Source: CAD feature listing. Evaluate the final solid. Frame: model axes, mm. Face numbers are marked on the shaded views. A direction names the side the tool comes from. Round coordinates to 2 decimals unless told otherwise and drop trailing zeros. Order: outer loops, then holes, each group sorted by start corner. A loop starts at its lowest first (then second) coordinate and runs counter-clockwise, first axis right, second up. Notation, with made-up numbers: M -33.5,-22.5 L 1.5,-22.5 A28 ccw 1.5,16.5 Z; hole C 58.5,61.5 d6. An arc over 180 degrees is marked long. Use one line per item in the form item = value. Start each with the question number.
Q1. Pull-direction query (X, two-part tool) for the marked faces 3, 4 and 5; classes: pulls with the +X half, pulls with the -X half, needs draft (parallel to the pull), parting line crosses it, or undercut.
Q2. Section C-C (z = 72). Return the cut outline in (x, y).
Q3. Material intervals for probe 1 along X at (y, z) = (-59.5, 29); probe 2 along Y at (x, z) = (-11, 73.5); probe 3 along Z at (x, y) = (16, 6.5), sorted ascending.
Q4. Section A-A (z = 35). Return the cut outline in (x, y), plus the area to 4 significant figures.
Q5. Section D-D (y = -66). Return the cut outline in (x, z), plus the area to 3 significant figures.
Q6. Contact query for flat-ended pins moving along their axis: pin 1 (8 mm diameter, centred on x = 0, z = 64.5, fed in from +Y); pin 2 (4 mm diameter, centred on x = 7.5, y = -67, fed in from -Z). Output: stop coordinate, or through.
Q7. Section B-B (y = -25.5). Return the cut outline in (x, z), plus the area to 4 significant figures.
Q8. Reachability of the marked faces 1 and 2 from +Z, -Z, +X, -X, +Y, -Y: full face, straight path, thin tool, end or side. Return the list, or none.
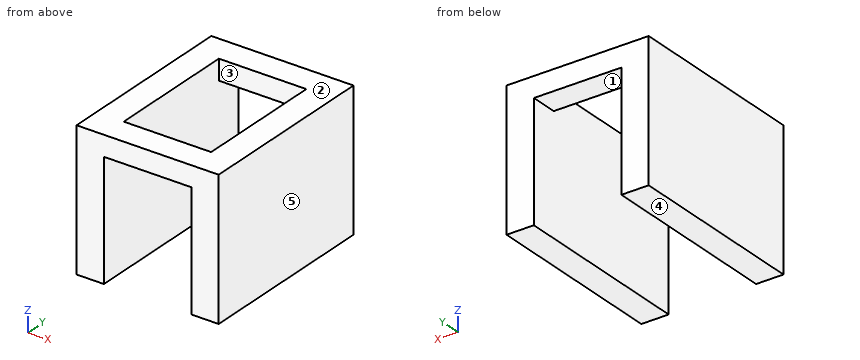
from build123d import *

# Parameters (mm, degrees)
SKETCH021_W     = 65
SKETCH021_H     = 85
PAD015_DEPTH    = 63
SKETCH022_W     = 40
SKETCH022_H     = 85
POCKET009_DEPTH = 53.7
SKETCH024_W     = 40
SKETCH024_H     = 60
POCKET010_DEPTH = 63


with BuildPart() as part:
    # Sketch021 → Pad015 (new body)
    with BuildSketch(Plane.XY):
        with Locations((0, -30)):
            Rectangle(SKETCH021_W, SKETCH021_H)
    extrude(amount=PAD015_DEPTH)

    # Sketch022 (on Face5 of Pad015) → Pocket009 (cut)
    with BuildSketch(Plane(origin=(0, 0, 0), x_dir=(1, 0, 0), z_dir=(0, 0, -1))):
        with Locations((0, 30)):
            Rectangle(SKETCH022_W, SKETCH022_H)
    extrude(amount=-POCKET009_DEPTH, mode=Mode.SUBTRACT)

    # Sketch024 → Pocket010 (cut)
    with BuildSketch(Plane.XY):
        with Locations((0, -30)):
            Rectangle(SKETCH024_W, SKETCH024_H)
    extrude(amount=POCKET010_DEPTH, mode=Mode.SUBTRACT)


with BuildPart() as part_1:
    # Body003 placement: moved
    add(part.part.moved(Location((0, 0, 15))))


solid = part_1.part
Results list:
q1.face_3 = undercut
q1.face_4 = needs draft
q1.face_5 = pulls with the +X half
q2.outline = M -32.5,-72.5 L 32.5,-72.5 L 32.5,12.5 L -32.5,12.5 Z; hole M -20,-60 L 20,-60 L 20,0 L -20,0 Z
q3.probe_1 = -32.5 to -20, 20 to 32.5
q3.probe_2 = -72.5 to -60, 0 to 12.5
q3.probe_3 = 68.7 to 78
q4.outline = M -32.5,-72.5 L -20,-72.5 L -20,12.5 L -32.5,12.5 Z; M 20,-72.5 L 32.5,-72.5 L 32.5,12.5 L 20,12.5 Z
q4.area = 2,125 mm2
q5.outline = M -32.5,15 L -20,15 L -20,68.7 L 20,68.7 L 20,15 L 32.5,15 L 32.5,78 L -32.5,78 Z
q5.area = 1,950 mm2
q6.pin_1 = through
q6.pin_2 = 68.7
q7.outline = M -32.5,15 L -20,15 L -20,78 L -32.5,78 Z; M 20,15 L 32.5,15 L 32.5,78 L 20,78 Z
q7.area = 1,575 mm2
q8.face_1 = -Z, +Y, -Y
q8.face_2 = +Z, +X, -X, +Y, -Y
